Geometry: final body of the model. Coordinates: model frame, mm. Face numbers are marked on the shaded views. A direction names the side the tool comes from. Round coordinates to 2 decimals unless told otherwise and drop trailing zeros. Order: outer loops, then holes, each group sorted by start corner. A loop starts at its lowest first (then second) coordinate and runs counter-clockwise, first axis right, second up. Notation, with made-up numbers: (-29, 63.25) - (-23, 63.25) arc R15 ccw to (-23, 88.25) - close; hole circle Ø9 at (-37, -13.5). An arc over 180 degrees is marked (long way). Put each result on its own line as item: value. Start each with the question number.
(1) Access query for the marked faces 1, 2 and 3. Directions: +Z, -Z, +X, -X, +Y, -Y. A direction counts if a zero-diameter tool reaches every point of the face in a straight line with its end or side. Return the directions, or none.
(2) Section C-C (z = 4). Output: boundary loops of the cut face in (x, y), and give its area (3 significant figures).
(3) Section D-D (x = 0). Output: boundary loops of the cut face in (y, z), and give its area (3 significant figures).
(4) Material intervals for L1, parallel to Y at x = 17, z = 12.75; L2, parallel to Y at x = 14.5, z = 9.5; L3, parallel to X at y = -15, z = 23, sorted ascending. Write a range as [from, to].
(5) Pin query (flat end, axial travel): P1, Ø4, axis at y = -32.5, z = 11, coming from the +X side; P2, Ø12, axis at x = -14, z = 15.5, coming from the +Y side; P3, Ø8, axis at x = -7, z = 9, coming from the +Y side. Return the tip coordinate at first contact, or that it passes through.
(6) Section B-B (x = 17). Output: boundary loops of the cut face in (y, z).
(7) Section A-A (y = 1.5). Output: boundary loops of the cut face in (x, z).
(8) Pull-direction query (Y, two-part tool) for the marked faces 4, 5 and 6; classes: released by +Y, released by -Y, zero draft, split by the parting line, or undercut.
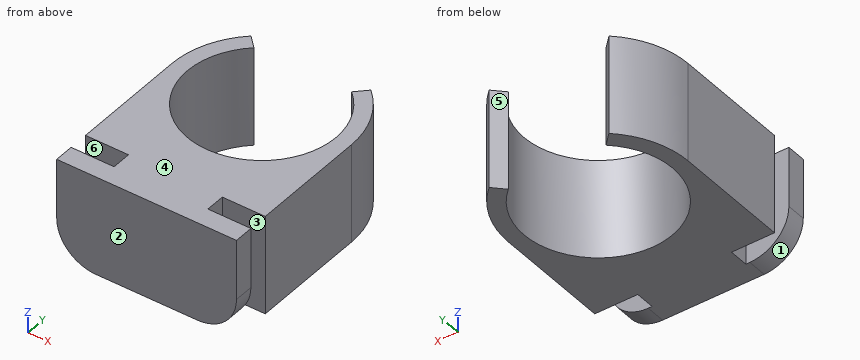
from build123d import *

# Parameters (mm, degrees)
F1_DEPTH = 25.4
F2_R     = 10
F3_R     = 10


with BuildPart() as f1:
    # F0 (on Top) → F1 (new body)
    with BuildSketch(Plane.XY):
        with BuildLine():
            ThreePointArc((12.5, 14.309088), (0, -19), (-12.5, 14.309088))
            Line((-12.5, 14.309088), (-15.333738, 17.142826))
            ThreePointArc((-15.333738, 17.142826), (-20.996142, 9.389463), (-23, 0))
            Line((-23, 0), (-23, -30))
            Line((-23, -30), (-12, -30))
            Line((-12, -30), (-12, -35))
            Line((-12, -35), (-23, -35))
            Line((-23, -35), (-23, -40))
            Line((-23, -40), (23, -40))
            Line((23, -40), (23, -35))
            Line((23, -35), (12, -35))
            Line((12, -35), (12, -30))
            Line((12, -30), (23, -30))
            Line((23, -30), (23, 0))
            ThreePointArc((23, 0), (20.996142, 9.389463), (15.333738, 17.142826))
            Line((15.333738, 17.142826), (12.5, 14.309088))
        make_face()
    extrude(amount=F1_DEPTH)

    # F2
    f2_edges = [f1.edges().sort_by_distance(p)[0] for p in [
        (23, -37.5, 0),
    ]]
    fillet(f2_edges, radius=F2_R)

    # F3
    f3_edges = [f1.edges().sort_by_distance(p)[0] for p in [
        (-23, -37.5, 0),
    ]]
    fillet(f3_edges, radius=F3_R)


solid = f1.part
Checks:
1. face 1: -Z, -X, -Y
1. face 2: +Z, -Z, +X, -X, -Y
1. face 3: +Z, -Z, +X
2. outline: (-23, -30) - (-12, -30) - (-12, -35) - (-21, -35) - (-21, -40) - (21, -40) - (21, -35) - (12, -35) - (12, -30) - (23, -30) - (23, 0) arc R23 ccw to (15.33, 17.14) - (12.5, 14.31) arc R19 cw (long way) to (-12.5, 14.31) - (-15.33, 17.14) arc R23 ccw to (-23, 0) - close
2. area: 1,290 mm²
3. outline: (-40, 0) - (-19, 0) - (-19, 25.4) - (-40, 25.4) - close
3. area: 533 mm²
4. L1: y = [-40, -35], [-30, -8.49], [8.49, 15.49]
4. L2: y = [-40, -35], [-30, -12.28], [12.28, 16.31]
4. L3: x = [-23, -11.66], [11.66, 23]
5. P1: stops at x = 12
5. P2: stops at y = 17.14
5. P3: stops at y = -15.49
6. outline: (-40, 0.83) - (-35, 0.83) - (-35, 25.4) - (-40, 25.4) - close; (-30, 0) - (-8.49, 0) - (-8.49, 25.4) - (-30, 25.4) - close; (8.49, 0) - (15.49, 0) - (15.49, 25.4) - (8.49, 25.4) - close
7. outline: (-22.95, 0) - (-18.94, 0) - (-18.94, 25.4) - (-22.95, 25.4) - close; (18.94, 0) - (22.95, 0) - (22.95, 25.4) - (18.94, 25.4) - close
8. face 4: zero draft
8. face 5: released by +Y
8. face 6: undercut
